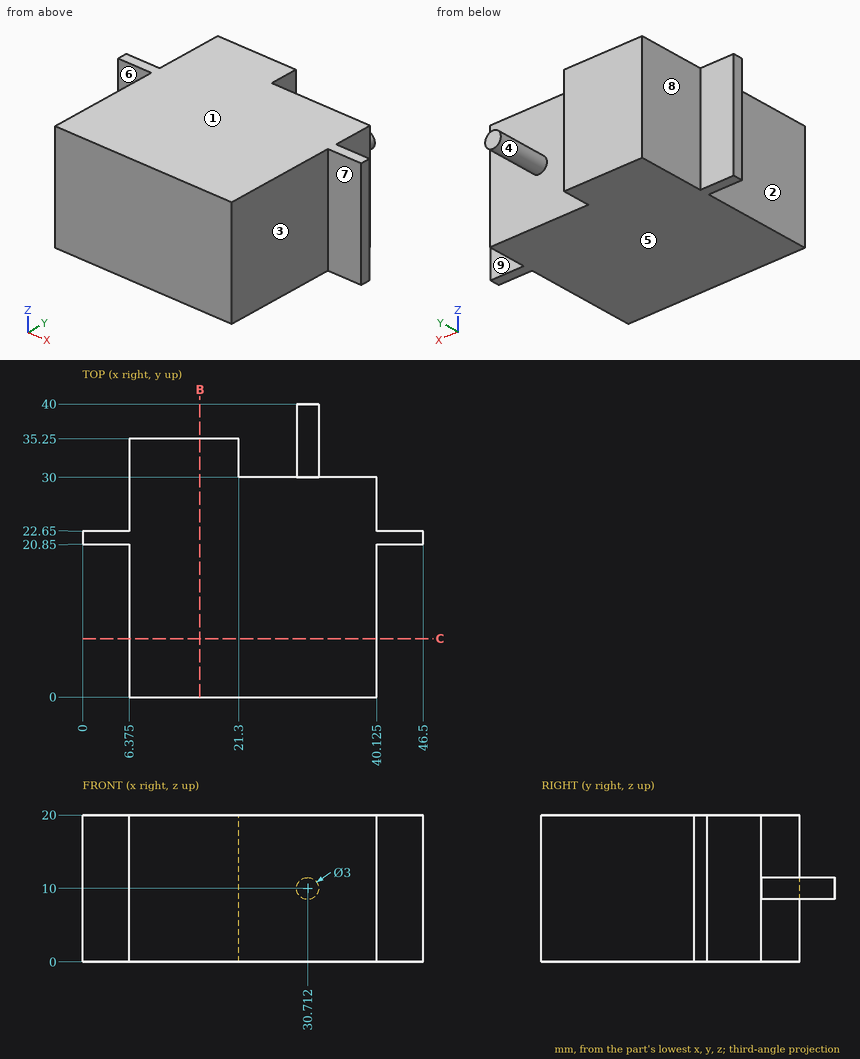
Geometry: see drawing. Coordinates: mm, zero at the bounding-box minimum. A direction names the side the tool comes from. Round coordinates to 2 decimals unless told otherwise and drop trailing zeros. Loops run counter-clockwise (first coordinate to the right, second up) from the corner with the lowest first, then second, coordinate; pieces in that order, holes last. Notation, with made-up numbers: (63, 11.25) -> (96, 11.25) arc R7 cw to (96, 21.25) -> close; hole circle Ø1 at (73.25, -10.5). An arc over 180 degrees is marked (long way). Write each question's results on one line, items separated by ' | '.
Item 1: Pull-direction query (X, two-part tool) for the marked faces 1, 2, 3 and 4; classes: pulls with the +X half, pulls with the -X half, needs draft (parallel to the pull), parting line crosses it, or undercut.
Answers below:
face 1: needs draft | face 2: pulls with the -X half | face 3: pulls with the +X half | face 4: undercut
Item 2: Pin query (flat end, axial travel): pin 1 Ø2 at (y, z) = (26, 13.5) entering from +X (1 decimal); pin 2 Ø5 at (x, y) = (40.5, 30.5) entering from -Z; pin 3 Ø3 at (x, z) = (42.5, 13.5) entering from -Y; pin 4 Ø5 at (x, z) = (43, 9) entering from +Y. Return the tip coordinate at first contact, or that it passes through.
Answers below:
pin 1: stops at x = 40.1 | pin 2: stops at z = 0 | pin 3: stops at y = 20.85 | pin 4: stops at y = 22.65
Item 3: Cut plane B-B on x = 16. Return the cut outline in (y, z), and give its area (3 significant figures).
Answers below:
outline: (0, 0) -> (35.25, 0) -> (35.25, 20) -> (0, 20) -> close | area: 705 mm²
Item 4: Cut plane C-C on y = 8. Return the cut outline in (x, z) (1 decimal).
Answers below:
outline: (6.4, 0) -> (40.1, 0) -> (40.1, 20) -> (6.4, 20) -> close
Item 5: Set-up query: the marked faces 5, 6, 7, 8 and 9. Return all of +Z, -Z, +X, -X, +Y, -Y with unobstructed straight access to the full face (end or side cutting, diameter ignored); none if empty.
Answers below:
face 5: -Z, +X, -X, +Y, -Y | face 6: +Z, -Z, -X, -Y | face 7: +Z, -Z, +X, -Y | face 8: +Z, -Z, -X, +Y | face 9: +Z, -Z, +X, +Y
Item 6: Line query: probe 1 along X at (y, z) = (28.5, 18) (1 decimal); probe 2 along Y at (x, z) = (32, 3.5); probe 3 along X at (y, z) = (31, 9.75) (1 decimal). Output: solid intervals per line, ascending. Write a range as [from, to].
Answers below:
probe 1: x = [6.4, 40.1] | probe 2: y = [0, 30] | probe 3: x = [6.4, 21.3], [29.2, 32.2]
